The model under review builds one solid part; all positions refer to its coordinate system, in mm. A direction names the side the tool comes from. Round coordinates to 2 decimals unless told otherwise and drop trailing zeros. Order: outer loops, then holes, each group sorted by start corner. A loop starts at its lowest first (then second) coordinate and runs counter-clockwise, first axis right, second up. Notation, with made-up numbers: M -40,15.5 L -11,15.5 A18 ccw -11,28.5 Z; hole C -19.75,17.5 d10. An arc over 180 degrees is marked long. Answer as a JSON object with one key per item and string values. Group by question number.
1) Consider section B-B, the plane y = 2. Write out the cut boundary in (x, z).
2) Insertion check: pin 1 Ø0.5 at (x, z) = (0.5, 0.5) entering from +Y; pin 2 Ø1.5 at (y, z) = (-0.5, 37) entering from +X; pin 3 Ø0.7 at (x, z) = (-0.5, 0.5) entering from +Y. Each pin has a flat end and moves straight along its axis. Give the tip position at first contact, or say it passes through.
3) Consider section A-A, the plane z = 4. Write out the cut boundary in (x, y).
4) The part is to be moulded in two halves that separate along X. For faces 3 (the flat face through (0, 0, 47.2)), 4 (the flat face through (2.75, 0, 1)), 5 (the flat face through (0, 0, 1)), 6 (the flat face through (-1.36, 2.39, 1.08)), say which applies: +X half, -X half, draft (parallel to the pull), parting line (faces both ways), or undercut.
5) Consider section C-C, the plane y = -2.25. Write out the cut boundary in (x, z), then the cut area to 3 significant figures.
6) For faces 1 (the flat face through (-1.394, -2.37, 1.085)), 2 (the cylindrical face through (-1.5, 0.07, 24.38)), list the 3-axis set-ups (+Z, -Z, +X, -X, +Y, -Y) from which the entire face can be reached by the end or side of a thin tool; tool diameter is ignored.
7) To check wall thickness, follow line 1 (Z direction, x = -0.7, y = -2.25); line 2 (Y direction, x = 1.2, z = 34.5); line 3 (X direction, y = -0.5, z = 27). State the ranges of each line that lie inside material, in increasing order.
```python
from build123d import *

# Parameters (mm, degrees)
SKETCH_1_R               = 1.5
EXTRUDE_3_DEPTH          = 2.2
SKETCH_1_6_R             = 1.5
EXTRUDE_4_DEPTH          = 47.2
CUT_EXTRUDE_1_DEPTH      = 1
CUT_EXTRUDE_1_DEPTH_BACK = 1


with BuildPart() as part:
    # Sketch 1 → Extrude 3 (new body)
    with BuildSketch(Plane.XY):
        Polygon((-2.75, 1.58771324), (-2.75, -1.58771324), (0, -3.175426481), (2.75, -1.58771324), (2.75, 1.58771324), (0, 3.175426481), align=None)
        Circle(SKETCH_1_R, mode=Mode.SUBTRACT)
    extrude(amount=EXTRUDE_3_DEPTH)

    # Sketch 1_6 → Extrude 4 (add)
    # profile 1 of 2: a face of its own
    with BuildSketch(Plane.XY):
        Circle(SKETCH_1_6_R)
        Polygon((-0.249002884, -0.902887914), (-0.249002884, -0.249002884), (-0.902887914, -0.249002884), (-0.902887914, 0.249002884), (-0.249002884, 0.249002884), (-0.249002884, 0.902887914), (0.249002884, 0.902887914), (0.249002884, 0.249002884), (0.902887914, 0.249002884), (0.902887914, -0.249002884), (0.249002884, -0.249002884), (0.249002884, -0.902887914), align=None, mode=Mode.SUBTRACT)
    # profile 2 of 2: a face of its own
    with BuildSketch(Plane.XY):
        Polygon((-0.249002884, -0.249002884), (-0.902887914, -0.249002884), (-0.902887914, 0.249002884), (-0.249002884, 0.249002884), (-0.249002884, 0.902887914), (0.249002884, 0.902887914), (0.249002884, 0.249002884), (0.902887914, 0.249002884), (0.902887914, -0.249002884), (0.249002884, -0.249002884), (0.249002884, -0.902887914), (-0.249002884, -0.902887914), align=None)
    extrude(amount=EXTRUDE_4_DEPTH)

    # Sketch 1_9 → Cut-Extrude 1 (cut, two sides: drawn at the far end of the back side and taken through both)
    with BuildSketch(Plane.XY.offset(-CUT_EXTRUDE_1_DEPTH_BACK)):
        Polygon((-0.249002884, -0.249002884), (-0.902887914, -0.249002884), (-0.902887914, 0.249002884), (-0.249002884, 0.249002884), (-0.249002884, 0.902887914), (0.249002884, 0.902887914), (0.249002884, 0.249002884), (0.902887914, 0.249002884), (0.902887914, -0.249002884), (0.249002884, -0.249002884), (0.249002884, -0.902887914), (-0.249002884, -0.902887914), align=None)
    extrude(amount=CUT_EXTRUDE_1_DEPTH + CUT_EXTRUDE_1_DEPTH_BACK, mode=Mode.SUBTRACT)


solid = part.part
```
Results list:
{
 "1": {"outline": "M -2.04,0 L 2.04,0 L 2.04,2.2 L -2.04,2.2 Z"},
 "2": {"pin 1": "y = 3.03", "pin 2": "x = 1.5", "pin 3": "y = 3.09"},
 "3": {"outline": "C 0,0 d3"},
 "4": {"face 3": "draft", "face 4": "+X half", "face 5": "undercut", "face 6": "-X half"},
 "5": {"outline": "M -1.6,0 L 1.6,0 L 1.6,2.2 L -1.6,2.2 Z", "area": "7.05 mm^2"},
 "6": {"face 1": "+Z, -Z, -X, -Y", "face 2": "+Z"},
 "7": {"line 1": "0 to 2.2", "line 2": "-0.9 to 0.9", "line 3": "-1.41 to 1.41"}
}
